Here's how the part is built. I have some questions about the finished solid (model axes, mm). Face numbers are marked on the shaded views. A direction names the side the tool comes from. Round coordinates to 2 decimals unless told otherwise and drop trailing zeros. One line per item, written item: value. Start each with the question number.
```python
from build123d import *

# Parameters (mm, degrees)
CUT_EXTRUDE_START        = 16.5
CUT_EXTRUDE_1_DEPTH      = 14
PATTERN_CIRCULAR_1_COUNT = 14
SKETCH_6_R               = 7
CUT_EXTRUDE_2_DEPTH      = 39.897300678
CHAMFER_1_SIZE           = 0.24
SKETCH_8_W               = 4
SKETCH_8_H               = 9
SKETCH_8_3_W             = 4
SKETCH_8_3_H             = 9


with BuildPart() as part:
    # 草图3 → 旋转1 (revolve)
    with BuildSketch(Plane.XY):
        Polygon((0, 0), (0, 17.54), (0.46, 18), (2.5, 18), (2.5, 20.84), (16.5, 20.84), (16.5, 18), (18.54, 18), (19, 17.54), (19, 0), align=None)
    revolve(axis=Axis((19, 0, 0), (-1, 0, 0)))

    # 草图4 → Cut-Extrude 1 (cut)
    with BuildSketch(Plane(origin=(0, 0, 0), x_dir=(0, 0, -1), z_dir=(1, 0, 0)).offset(CUT_EXTRUDE_START)):
        with BuildLine():
            Line((-0.947821517, 18.71), (0.947821517, 18.71))
            ThreePointArc((0.947821517, 18.71), (1.441097252, 18.865529242), (1.755957171, 19.275862677))
            Line((1.755957171, 19.275862677), (2.135902122, 20.319752849))
            ThreePointArc((2.135902122, 20.319752849), (2.358797616, 20.591469041), (2.702673222, 20.664006326))
            ThreePointArc((2.702673222, 20.664006326), (0, 20.84), (-2.702673222, 20.664006326))
            ThreePointArc((-2.702673222, 20.664006326), (-2.358797616, 20.591469041), (-2.135902122, 20.319752849))
            Line((-2.135902122, 20.319752849), (-1.755957171, 19.275862677))
            ThreePointArc((-1.755957171, 19.275862677), (-1.441097252, 18.865529242), (-0.947821517, 18.71))
        make_face()
    cut_extrude_1 = extrude(amount=-CUT_EXTRUDE_1_DEPTH, mode=Mode.SUBTRACT)

    # 阵列(圆周)1: Cut-Extrude 1 ×14 about axis
    pattern_circular_1_axis = Axis((0, 0, 0), (1, 0, 0))
    for i in range(1, PATTERN_CIRCULAR_1_COUNT):
        add(cut_extrude_1.rotate(pattern_circular_1_axis, i * 360 / PATTERN_CIRCULAR_1_COUNT), mode=Mode.SUBTRACT)

    # 草图5 → 旋转2 (revolve)
    with BuildSketch(Plane.XY, mode=Mode.PRIVATE) as revolve_2_sk:
        Polygon((1.9, 24), (2.5, 20.84), (2.5, 18), (1, 18), (1, 20.84), (0.4, 24), align=None)
        Polygon((18, 18), (16.5, 18), (16.5, 20.84), (17.1, 24), (18.6, 24), (18, 20.84), align=None)
    revolve(revolve_2_sk.sketch.rotate(Axis((0, 0, 0), (1, 0, 0)), 180), axis=Axis((0, 0, 0), (1, 0, 0)))

    # 草图6 → 切除-拉伸2 (cut, through all)
    with BuildSketch(Plane(origin=(0, 0, 0), x_dir=(0, 0, -1), z_dir=(1, 0, 0))):
        Circle(SKETCH_6_R)
    extrude(amount=CUT_EXTRUDE_2_DEPTH, mode=Mode.SUBTRACT)

    # 倒角1
    chamfer_1_edges = [part.edges().sort_by_distance(p)[0] for p in [
        (0, 0, 7),
        (19, 0, 7),
    ]]
    chamfer(chamfer_1_edges, length=CHAMFER_1_SIZE)

    # 草图8 → 旋转3 (revolve)
    with BuildSketch(Plane.XY, mode=Mode.PRIVATE) as revolve_3_sk:
        with Locations((1, 4.5)):
            Rectangle(SKETCH_8_W, SKETCH_8_H)
    revolve(revolve_3_sk.sketch.rotate(Axis((-1, 0, 0), (1, 0, 0)), 90), axis=Axis((-1, 0, 0), (1, 0, 0)))

    # 草图8<3> → 切除-旋转4 (revolve, cut)
    with BuildSketch(Plane.XY, mode=Mode.PRIVATE) as cut_revolve_4_sk:
        with Locations((1, 4.5)):
            Rectangle(SKETCH_8_3_W, SKETCH_8_3_H)
    revolve(cut_revolve_4_sk.sketch.rotate(Axis((-1, 0, 0), (1, 0, 0)), 90), axis=Axis((-1, 0, 0), (1, 0, 0)), mode=Mode.SUBTRACT)


solid = part.part
```
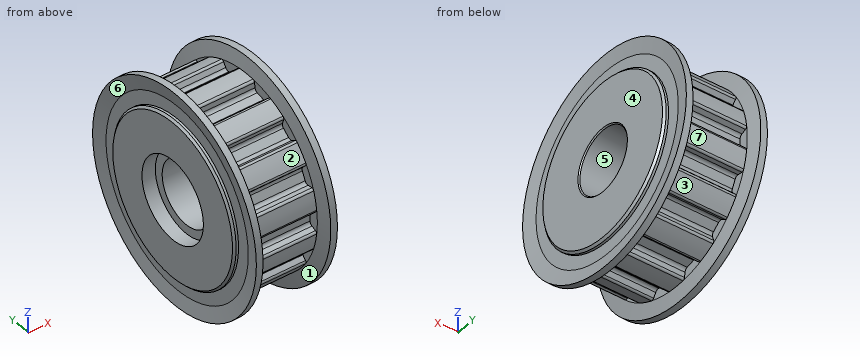
Q1. If I drill on line 1 along Z through (x, y) = (15.25, 0); line 2 along Y through (x, z) = (14.5, 0); line 3 along Y through (x, z) = (4.5, 11), over which ranges is the centre line in solid material (lowest first)?
Q2. Which directions (+Z, -Z, +X, -X, +Y, -Y) give clear straight access to the entire face, cutting with the end or side of a thin tool? Please do the marked faces 1, 2 and 3.
Q3. Will these pins go through, and if not, where does the flat tip stop? P1, Ø4, axis at x = 10, z = -4.5, coming from the +Y side; P2, Ø1.7, axis at y = 20, z = 0, coming from the +X side; P3, Ø3, axis at y = -19, z = 4, coming from the -X side; P4, Ø20, axis at y = -1, z = 2, coming from the -X side.
Q4. If we mould it in two halves opening along X, with no side actions, what happens to the marked faces 4, 5, 6 and 7? For each: released by +X, released by -X, zero draft, split by the parting line, or undercut.
Answers below:
1. line 1: z = -20.84 to -7, 7 to 20.84
1. line 2: y = -18.71 to -7, 7 to 18.71
1. line 3: y = -17.52 to 17.52
2. face 1: none
2. face 2: +Z, -Y
2. face 3: -Z, +Y
3. P1: stops at y = 20.67
3. P2: stops at x = 18
3. P3: stops at x = 0.38
3. P4: stops at x = 0
4. face 4: released by +X
4. face 5: zero draft
4. face 6: released by -X
4. face 7: undercut
